```python
from build123d import *

# Parameters (mm, degrees)
SKETCH2_R           = 6
SKETCH2_R_2         = 1.5
BOSS_EXTRUDE1_DEPTH = 1.15
SKETCH3_R           = 4.4
BOSS_EXTRUDE2_DEPTH = 3.2
SKETCH4_R           = 0.75
BOSS_EXTRUDE3_DEPTH = 1.15


with BuildPart() as part:
    # Sketch2 → Boss-Extrude1 (new, symmetric)
    with BuildSketch(Plane(origin=(0, 0, 0), x_dir=(1, 0, 0), z_dir=(0, 1, 0))):
        with Locations(Location((0, 0, 0), (0, 0, 270))):
            Circle(SKETCH2_R)
        with Locations(Location((0, 0, 0), (0, 0, 270))):
            Circle(SKETCH2_R_2, mode=Mode.SUBTRACT)
    extrude(amount=BOSS_EXTRUDE1_DEPTH, both=True)

    # Sketch3 → Boss-Extrude2 (add)
    with BuildSketch(Plane(origin=(0, 1.15, 0), x_dir=(1, 0, 0), z_dir=(0, 1, 0))):
        with Locations(Location((0, 0, 0), (0, 0, 270))):
            Circle(SKETCH3_R)
        with BuildLine():
            Line((0.107421435, 2.898009771), (0.338399731, 2.678709694))
            Line((0.338399731, 2.678709694), (0.61665913, 2.83367809))
            ThreePointArc((0.61665913, 2.83367809), (0.721200673, 2.808891167), (0.824752316, 2.780248841))
            Line((0.824752316, 2.780248841), (0.993936292, 2.510396512))
            Line((0.993936292, 2.510396512), (1.301992734, 2.591295993))
            ThreePointArc((1.301992734, 2.591295993), (1.397085655, 2.541289372), (1.490260976, 2.48779465))
            Line((1.490260976, 2.48779465), (1.587020181, 2.184345885))
            Line((1.587020181, 2.184345885), (1.905517346, 2.186093238))
            ThreePointArc((1.905517346, 2.186093238), (1.985186607, 2.11400902), (2.062131058, 2.039023173))
            Line((2.062131058, 2.039023173), (2.080385755, 1.721044772))
            Line((2.080385755, 1.721044772), (2.389311295, 1.643530205))
            ThreePointArc((2.389311295, 1.643530205), (2.448550984, 1.553897705), (2.504429862, 1.46213237))
            Line((2.504429862, 1.46213237), (2.443033042, 1.149604087))
            Line((2.443033042, 1.149604087), (2.722976028, 0.997698125))
            ThreePointArc((2.722976028, 0.997698125), (2.758063897, 0.896149284), (2.789366126, 0.793370413))
            Line((2.789366126, 0.793370413), (2.652175577, 0.505929549))
            Line((2.652175577, 0.505929549), (2.885546163, 0.289177003))
            ThreePointArc((2.885546163, 0.289177003), (2.894277512, 0.182092507), (2.899036259, 0.074758075))
            Line((2.899036259, 0.074758075), (2.694672167, -0.169534403))
            Line((2.694672167, -0.169534403), (2.866806821, -0.437514174))
            ThreePointArc((2.866806821, -0.437514174), (2.848633027, -0.543405812), (2.826549281, -0.648551587))
            Line((2.826549281, -0.648551587), (2.567852594, -0.834345885))
            Line((2.567852594, -0.834345885), (2.667935462, -1.136714727))
            ThreePointArc((2.667935462, -1.136714727), (2.623998452, -1.234759946), (2.576459817, -1.331110368))
            Line((2.576459817, -1.331110368), (2.279685399, -1.446732346))
            Line((2.279685399, -1.446732346), (2.301427906, -1.764491312))
            ThreePointArc((2.301427906, -1.764491312), (2.234488404, -1.84852957), (2.164481907, -1.930030589))
            Line((2.164481907, -1.930030589), (1.848277186, -1.968215294))
            Line((1.848277186, -1.968215294), (1.790313171, -2.281398419))
            ThreePointArc((1.790313171, -2.281398419), (1.704577232, -2.346149284), (1.616501638, -2.40767989))
            Line((1.616501638, -2.40767989), (1.30073492, -2.366028036))
            Line((1.30073492, -2.366028036), (1.166706475, -2.654956874))
            ThreePointArc((1.166706475, -2.654956874), (1.067561203, -2.696351809), (0.966950626, -2.734045809))
            Line((0.966950626, -2.734045809), (0.671462695, -2.615174535))
            Line((0.671462695, -2.615174535), (0.469791321, -2.861694623))
            ThreePointArc((0.469791321, -2.861694623), (0.363466377, -2.877132634), (0.25664255, -2.888621575))
            Line((0.25664255, -2.888621575), (0, -2.7))
            Line((0, -2.7), (-0.25664255, -2.888621575))
            ThreePointArc((-0.25664255, -2.888621575), (-0.363466377, -2.877132634), (-0.469791321, -2.861694623))
            Line((-0.469791321, -2.861694623), (-0.671462695, -2.615174535))
            Line((-0.671462695, -2.615174535), (-0.966950626, -2.734045809))
            ThreePointArc((-0.966950626, -2.734045809), (-1.067561203, -2.696351809), (-1.166706475, -2.654956874))
            Line((-1.166706475, -2.654956874), (-1.30073492, -2.366028036))
            Line((-1.30073492, -2.366028036), (-1.616501638, -2.40767989))
            ThreePointArc((-1.616501638, -2.40767989), (-1.704577232, -2.346149284), (-1.790313171, -2.281398419))
            Line((-1.790313171, -2.281398419), (-1.848277186, -1.968215294))
            Line((-1.848277186, -1.968215294), (-2.164481907, -1.930030589))
            ThreePointArc((-2.164481907, -1.930030589), (-2.234488404, -1.84852957), (-2.301427906, -1.764491312))
            Line((-2.301427906, -1.764491312), (-2.279685399, -1.446732346))
            Line((-2.279685399, -1.446732346), (-2.576459817, -1.331110368))
            ThreePointArc((-2.576459817, -1.331110368), (-2.623998452, -1.234759946), (-2.667935462, -1.136714727))
            Line((-2.667935462, -1.136714727), (-2.567852594, -0.834345885))
            Line((-2.567852594, -0.834345885), (-2.826549281, -0.648551587))
            ThreePointArc((-2.826549281, -0.648551587), (-2.848633027, -0.543405812), (-2.866806821, -0.437514174))
            Line((-2.866806821, -0.437514174), (-2.694672167, -0.169534403))
            Line((-2.694672167, -0.169534403), (-2.899036259, 0.074758075))
            ThreePointArc((-2.899036259, 0.074758075), (-2.894277512, 0.182092507), (-2.885546163, 0.289177003))
            Line((-2.885546163, 0.289177003), (-2.652175577, 0.505929549))
            Line((-2.652175577, 0.505929549), (-2.789366126, 0.793370413))
            ThreePointArc((-2.789366126, 0.793370413), (-2.758063897, 0.896149284), (-2.722976028, 0.997698125))
            Line((-2.722976028, 0.997698125), (-2.443033042, 1.149604087))
            Line((-2.443033042, 1.149604087), (-2.504429862, 1.46213237))
            ThreePointArc((-2.504429862, 1.46213237), (-2.448550984, 1.553897705), (-2.389311295, 1.643530205))
            Line((-2.389311295, 1.643530205), (-2.080385755, 1.721044772))
            Line((-2.080385755, 1.721044772), (-2.062131058, 2.039023173))
            ThreePointArc((-2.062131058, 2.039023173), (-1.985186607, 2.11400902), (-1.905517346, 2.186093238))
            Line((-1.905517346, 2.186093238), (-1.587020181, 2.184345885))
            Line((-1.587020181, 2.184345885), (-1.490260976, 2.48779465))
            ThreePointArc((-1.490260976, 2.48779465), (-1.397085655, 2.541289372), (-1.301992734, 2.591295993))
            Line((-1.301992734, 2.591295993), (-0.993936292, 2.510396512))
            Line((-0.993936292, 2.510396512), (-0.824752316, 2.780248841))
            ThreePointArc((-0.824752316, 2.780248841), (-0.721200673, 2.808891167), (-0.61665913, 2.83367809))
            Line((-0.61665913, 2.83367809), (-0.338399731, 2.678709694))
            Line((-0.338399731, 2.678709694), (-0.107421435, 2.898009771))
            ThreePointArc((-0.107421435, 2.898009771), (0, 2.9), (0.107421435, 2.898009771))
        make_face(mode=Mode.SUBTRACT)
    extrude(amount=BOSS_EXTRUDE2_DEPTH)

    # Sketch4 → Boss-Extrude3 (add, symmetric)
    with BuildSketch(Plane(origin=(0, 0, 0), x_dir=(1, 0, 0), z_dir=(0, 1, 0))):
        with BuildLine():
            Line((3.968626967, 4.5), (16.888114198, 2.469689731))
            ThreePointArc((16.888114198, 2.469689731), (19, 0), (16.888114198, -2.469689731))
            Line((16.888114198, -2.469689731), (3.968626967, -4.5))
            ThreePointArc((3.968626967, -4.5), (6, 0), (3.968626967, 4.5))
        make_face()
        with Locations(Location((16, 0, 0), (0, 0, 270))):
            Circle(SKETCH4_R, mode=Mode.SUBTRACT)
        with Locations(Location((13, 0, 0), (0, 0, 270))):
            Circle(SKETCH4_R, mode=Mode.SUBTRACT)
        with Locations(Location((10, 0, 0), (0, 0, 270))):
            Circle(SKETCH4_R, mode=Mode.SUBTRACT)
        with Locations(Location((7, 0, 0), (0, 0, 270))):
            Circle(SKETCH4_R, mode=Mode.SUBTRACT)
    extrude(amount=BOSS_EXTRUDE3_DEPTH, both=True)


solid = part.part
```
Geometry check sheet. Reference: the model listing, model coordinates, mm. A direction names the side the tool comes from. Round coordinates to 2 decimals unless told otherwise and drop trailing zeros. Write each loop counter-clockwise with the first axis right and the second up, starting at its lowest first coordinate (ties: lowest second). Pieces come first, ordered by that corner, then holes. Notation, with made-up numbers: (85, -29.5) - (121, -29.5) arc R14 ccw to (121, -11.5) - close; hole circle Ø11 at (74.25, 15.25). An arc over 180 degrees is marked (long way). Write each question's results on one line, items separated by ' | '.
(1) Depth check by flat-ended pin: pin 1 Ø3.5 at (x, z) = (10, -2) entering from +Y; pin 2 Ø3 at (y, z) = (3.5, -3.5) entering from +X; pin 3 Ø1.5 at (y, z) = (2.5, 1.5) entering from +X. Enter the tip coordinate at first touch or a pass-through.
Computed:
pin 1: stops at y = 1.15 | pin 2: stops at x = 3.92 | pin 3: stops at x = 4.34
(2) Sectioned sample at B-B, the plane x = 10. Enter the section's corners in (y, z), plus the area to 3 significant figures.
Computed:
outline: (-1.15, -3.55) - (1.15, -3.55) - (1.15, -0.75) - (-1.15, -0.75) - close; (-1.15, 0.75) - (1.15, 0.75) - (1.15, 3.55) - (-1.15, 3.55) - close | area: 12.9 mm^2
(3) Sectioned sample at C-C, the plane z = 3.25. Enter the section's corners in (x, y).
Computed:
outline: (-5.04, -1.15) - (11.92, -1.15) - (11.92, 1.15) - (2.97, 1.15) - (2.97, 4.35) - (-2.97, 4.35) - (-2.97, 1.15) - (-5.04, 1.15) - close
(4) Sectioned sample at D-D, the plane x = 7. Enter the section's corners in (y, z).
Computed:
outline: (-1.15, -4.02) - (1.15, -4.02) - (1.15, -0.75) - (-1.15, -0.75) - close; (-1.15, 0.75) - (1.15, 0.75) - (1.15, 4.02) - (-1.15, 4.02) - close
(5) Sectioned sample at A-A, the plane y = -0.4. Enter the section's corners in (x, z), plus the area to 3 significant figures.
Computed:
outline: (3.97, -4.5) - (16.89, -2.47) arc R2.5 ccw to (16.89, 2.47) - (3.97, 4.5) arc R6 ccw (long way) to start; hole circle Ø3 at (0, 0); hole circle Ø1.5 at (7, 0); hole circle Ø1.5 at (10, 0); hole circle Ø1.5 at (13, 0); hole circle Ø1.5 at (16, 0) | area: 184 mm^2
(6) Set-up check for faces 4 (the face through (10.52, 0.02, 3.47)), 5 (the face through (1.3, 1.15, 1.2)): record each of +Z, -Z, +X, -X, +Y, -Y from which the full face is reachable in a straight line by a thin tool's end or side.
Computed:
face 4: +Z, +X, +Y, -Y | face 5: +Y
(7) Draft check along X on faces 1 (the face through (0, 4.35, 3)), 2 (the face through (10.632, -0.016, 0.403)), 3 (the face through (19, 0, 0)). Enter one of: pulls with the +X half, pulls with the -X half, needs draft (parallel to the pull), parting line crosses it, or undercut.
Computed:
face 1: needs draft | face 2: undercut | face 3: pulls with the +X half
(8) Thickness scan on probe 1 along X at (y, z) = (-0.1, 0); probe 2 along Y at (x, z) = (4, 4.25); probe 3 along X at (y, z) = (1.85, 0). Record the ranges inside material, lowest first. Write a range as from..to.
Computed:
probe 1: x = -6..-1.5, 1.5..6.25, 7.75..9.25, 10.75..12.25, 13.75..15.25, 16.75..19 | probe 2: y = -1.15..1.15 | probe 3: x = -4.4..-2.84, 2.84..4.4
